Autodesk Inventor part; units mm, degrees
ref_plane "YZ Plane" through (0, 0, 0) normal (1, 0, 0) x (0, 1, 0)
ref_plane "XZ Plane" through (0, 0, 0) normal (0, 1, 0) x (-1, 0, 0)
ref_plane "XY Plane" through (0, 0, 0) normal (0, 0, 1) x (1, 0, 0)
sketch "Sketch1" plane through (0, 0, 0) normal (0, 0, 1) x (1, 0, 0)
  line L0 (-12.7, 12.7) -> (12.7, 12.7)
  line L1 (12.7, 12.7) -> (12.7, -12.7)
  line L2 (12.7, -12.7) -> (-12.7, -12.7)
  line L3 (-12.7, -12.7) -> (-12.7, 12.7)
  line L4 (9.652, 9.652) -> (-9.652, 9.652)
  line L5 (-9.652, 9.652) -> (-9.652, -9.652)
  line L6 (-9.652, -9.652) -> (9.652, -9.652)
  line L7 (9.652, -9.652) -> (9.652, 9.652)
  point P0 (0, 0)
  point P1 (12.7, 0)
  point P2 (0, 12.7)
  dimension "d0" = 25.4
  dimension "d1" = 25.4
  dimension "d2" = 3.048
extrude "Extrusion1" add sketch "Sketch1" along normal mid plane 1422.4
sketch "Sketch2" plane through (0, 0, 0) normal (0, 0, 1) x (1, 0, 0)
  point P0 (0, 0)
sketch "Sketch3" plane through (12.7, 12.7, 711.2) normal (1, 0, 0) x (0, 0, -1)
  circle A0 centre (1248.4758, -12.693) radius 4.25
  circle A1 centre (1168.4758, -12.693) radius 4.4
  circle A2 centre (253.9242, -12.693) radius 4.4
  circle A3 centre (173.9242, -12.693) radius 4.25
  point P0 (711.2, -12.7)
  point P1 (488.8742, -12.693)
  point P2 (374.5742, -12.693)
  point P3 (933.5258, -12.693)
  point P4 (1047.8258, -12.693)
  dimension "d5" = 114.3
  dimension "d6" = 120.65
  dimension "d7" = 120.65
  dimension "d8" = 114.3
hole "Hole1" at (12.7, 0.007, -537.2758) at (12.7, 0.007, -457.2758) at (12.7, 0.007, -336.6258) at (12.7, 0.007, -222.3258) at (12.7, 0.007, 222.3258) at (12.7, 0.007, 336.6258) at (12.7, 0.007, 457.2758) at (12.7, 0.007, 537.2758) direction (-1, 0, 0) diameter 6.7469 depth 3.175 tip angle 118
sketch "Sketch4" plane through (-12.7, -12.7, -711.2) normal (-1, 0, 0) x (0, 0, 1)
  circle A0 centre (173.9242, 12.707) radius 3.3734
  circle A1 centre (253.9242, 12.707) radius 3.3734
  circle A2 centre (374.5742, 12.707) radius 3.3734
  circle A3 centre (488.8742, 12.707) radius 3.3734
  circle A4 centre (933.5258, 12.707) radius 3.3734
  circle A5 centre (1047.8258, 12.707) radius 3.3734
  circle A6 centre (1168.4758, 12.707) radius 3.3734
  circle A7 centre (1248.4758, 12.707) radius 3.3734
  point P0 (711.2, 12.7)
hole "Hole2" at (-12.7, 0.007, 537.2758) at (-12.7, 0.007, 457.2758) at (-12.7, 0.007, 336.6258) at (-12.7, 0.007, 222.3258) at (-12.7, 0.007, -222.3258) at (-12.7, 0.007, -336.6258) at (-12.7, 0.007, -457.2758) at (-12.7, 0.007, -537.2758) direction (1, 0, 0) diameter 12.7 depth 3.175 tip angle 118
equation "\"d2\" = thick"
equation "\"d3\" = L2"
equation "\"L\" = 1219.2"
equation "\"thick\" = 3.048"
equation "\"L2\" = 1422.4"
properties part number "1inSquareSupportOut"
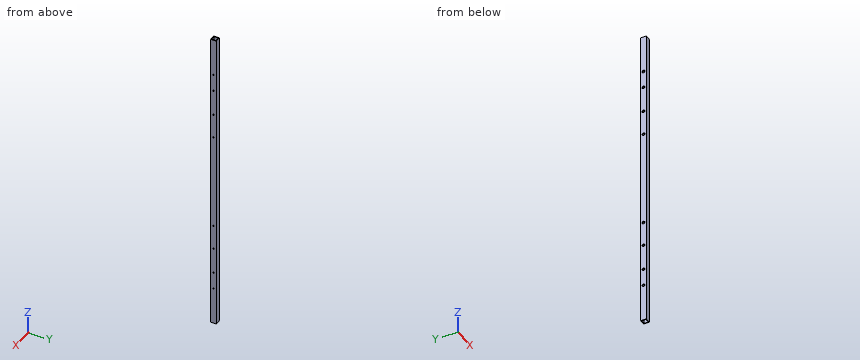
Could you check a few things on this model? Use its own coordinates, in mm. Round coordinates to 2 decimals unless told otherwise and drop trailing zeros. Loops run counter-clockwise (first coordinate to the right, second up) from the corner with the lowest first, then second, coordinate; pieces in that order, holes last. Notation, with made-up numbers: (21, 30) -> (69, 30) arc R25 cw to (69, 50) -> close; hole circle Ø3 at (51, -4). An arc over 180 degrees is marked (long way). One line per question, with ' | ' between items.
(1) If we section it at B-B on z = 385.5: List the corners of the cut face in (x, y) for me, and give its area (3 significant figures).
Model answer:
outline: (-12.7, -12.7) -> (12.7, -12.7) -> (12.7, 12.7) -> (-12.7, 12.7) -> close; hole (-9.65, -9.65) -> (9.65, -9.65) -> (9.65, 9.65) -> (-9.65, 9.65) -> close | area: 273 mm^2
(2) For pin 1 Ø9 at (y, z) = (0.01, 222.33) entering from -X, with a flat end and sliding along its axis, tell me the tip position at first contact or that it passes through.
Model answer:
pin 1: stops at x = 9.65
(3) If we section it at A-A on x = -3.5: List the corners of the cut face in (y, z) for me, and give its area (3 significant figures).
Model answer:
outline: (-12.7, -711.2) -> (-9.65, -711.2) -> (-9.65, 711.2) -> (-12.7, 711.2) -> close; (9.65, -711.2) -> (12.7, -711.2) -> (12.7, 711.2) -> (9.65, 711.2) -> close | area: 8,670 mm^2
(4) If I drill on probe 1 along Y at (x, z) = (-2, 132), over which ranges is the centre line in solid material (lowest first)?
Model answer:
probe 1: y = -12.7 to -9.65, 9.65 to 12.7
